The listing builds one solid part. Answer for the finished solid, in the listing's coordinates (mm). Face numbers are marked on the shaded views. A direction names the side the tool comes from. Give positions to 0.01 mm unless a question says otherwise; leave off trailing zeros. Loops run counter-clockwise (first coordinate to the right, second up) from the corner with the lowest first, then second, coordinate; pieces in that order, holes last. Notation, with made-up numbers: (-26.75, 68.5) - (31.25, 68.5) arc R7 cw to (31.25, 80.5) - close; hole circle Ø2 at (-33, -21). An arc over 180 degrees is marked (long way). Write each question's results on one line, items separated by ' | '.
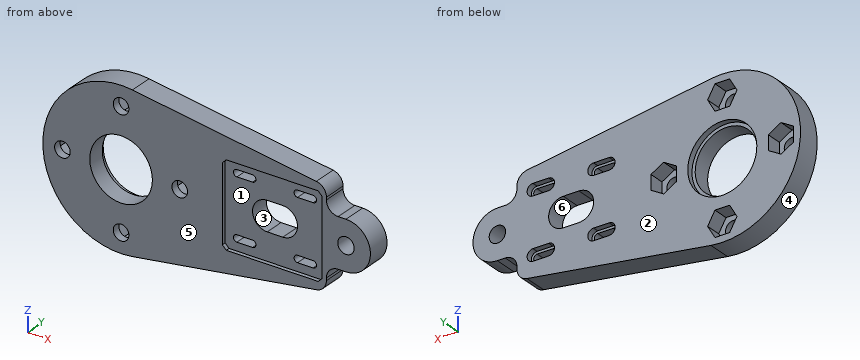
from build123d import *

# Parameters (mm, degrees)
SKETCH1_R           = 10
BOSS_EXTRUDE1_DEPTH = 12
SKETCH2_R           = 17.65
CUT_EXTRUDE1_DEPTH  = 3
CUT_EXTRUDE2_DEPTH  = 12
SKETCH4_R           = 4
CUT_EXTRUDE3_DEPTH  = 12
SKETCH5_R           = 16
CUT_EXTRUDE4_DEPTH  = 113.720894248
SKETCH6_W           = 51
SKETCH6_H           = 43
CUT_EXTRUDE5_DEPTH  = 2
CHAMFER1_SIZE       = 2
CUT_EXTRUDE6_DEPTH  = 8
CUT_EXTRUDE7_DEPTH  = 3
CUT_EXTRUDE8_DEPTH  = 7
SKETCH11_R          = 4.2
BOSS_EXTRUDE2_DEPTH = 12
FILLET1_R           = 6


with BuildPart() as part:
    # Sketch1 → Boss-Extrude1 (new body)
    with BuildSketch(Plane(origin=(0, 0, 0), x_dir=(1, 0, 0), z_dir=(0, 1, 0))):
        with BuildLine():
            Line((5.815477401, 39.574994916), (105, 25))
            Line((105, 25), (105, -25))
            Line((105, -25), (5.815477401, -39.574994916))
            ThreePointArc((5.815477401, -39.574994916), (-40, 0), (5.815477401, 39.574994916))
        make_face()
        with Locations(Location((0, 0, 0), (0, 0, 270))):
            Circle(SKETCH1_R, mode=Mode.SUBTRACT)
    extrude(amount=BOSS_EXTRUDE1_DEPTH)

    # Sketch2 → Cut-Extrude1 (cut)
    with BuildSketch(Plane(origin=(0, 12, 0), x_dir=(1, 0, 0), z_dir=(0, 1, 0))):
        with Locations(Location((0, 0, 0), (0, 0, 270))):
            Circle(SKETCH2_R)
    extrude(amount=-CUT_EXTRUDE1_DEPTH, mode=Mode.SUBTRACT)

    # Sketch3 → Cut-Extrude2 (cut)
    with BuildSketch(Plane(origin=(0, 12, 0), x_dir=(1, 0, 0), z_dir=(0, 1, 0))):
        with BuildLine():
            Line((73.3, 7.5), (81.3, 7.5))
            ThreePointArc((81.3, 7.5), (88.8, 0), (81.3, -7.5))
            Line((81.3, -7.5), (73.3, -7.5))
            ThreePointArc((73.3, -7.5), (65.8, 0), (73.3, 7.5))
        make_face()
    extrude(amount=-CUT_EXTRUDE2_DEPTH, mode=Mode.SUBTRACT)

    # Sketch4 → Cut-Extrude3 (cut)
    with BuildSketch(Plane(origin=(0, 12, 0), x_dir=(1, 0, 0), z_dir=(0, 1, 0))):
        with Locations(Location((30, 0, 0), (0, 0, 270))):
            Circle(SKETCH4_R)
        with Locations(Location((0, -30, 0), (0, 0, 270))):
            Circle(SKETCH4_R)
        with Locations(Location((-30, 0, 0), (0, 0, 270))):
            Circle(SKETCH4_R)
        with Locations(Location((0, 30, 0), (0, 0, 270))):
            Circle(SKETCH4_R)
    extrude(amount=-CUT_EXTRUDE3_DEPTH, mode=Mode.SUBTRACT)

    # Sketch5 → Cut-Extrude4 (cut, through all)
    with BuildSketch(Plane.XZ.offset(-9)):
        with Locations(Location((0, 0, 0), (0, 0, 270))):
            Circle(SKETCH5_R)
    extrude(amount=CUT_EXTRUDE4_DEPTH, mode=Mode.SUBTRACT)

    # Sketch6 → Cut-Extrude5 (cut)
    with BuildSketch(Plane.XZ):
        with Locations((77.3, 0)):
            Rectangle(SKETCH6_W, SKETCH6_H)
    extrude(amount=-CUT_EXTRUDE5_DEPTH, mode=Mode.SUBTRACT)

    # Chamfer1
    chamfer1_edges = [part.edges().sort_by_distance(p)[0] for p in [
        (102.8, 1, 21.5),
        (102.8, 1, -21.5),
        (51.8, 1, -21.5),
        (51.8, 1, 21.5),
    ]]
    chamfer(chamfer1_edges, length=CHAMFER1_SIZE)

    # Sketch7 → Cut-Extrude6 (cut)
    with BuildSketch(Plane(origin=(0, 12, 0), x_dir=(1, 0, 0), z_dir=(0, 1, 0))):
        Polygon((-7.505553499, 30), (-3.75277675, 23.5), (3.75277675, 23.5), (7.505553499, 30), (3.75277675, 36.5), (-3.75277675, 36.5), align=None)
        Polygon((-30, -7.505553499), (-23.5, -3.75277675), (-23.5, 3.75277675), (-30, 7.505553499), (-36.5, 3.75277675), (-36.5, -3.75277675), align=None)
        Polygon((30, 7.505553499), (23.5, 3.75277675), (23.5, -3.75277675), (30, -7.505553499), (36.5, -3.75277675), (36.5, 3.75277675), align=None)
        Polygon((7.505553499, -30), (3.75277675, -23.5), (-3.75277675, -23.5), (-7.505553499, -30), (-3.75277675, -36.5), (3.75277675, -36.5), align=None)
    extrude(amount=-CUT_EXTRUDE6_DEPTH, mode=Mode.SUBTRACT)

    # Sketch9 → Cut-Extrude7 (cut)
    with BuildSketch(Plane(origin=(0, 12, 0), x_dir=(1, 0, 0), z_dir=(0, 1, 0))):
        with BuildLine():
            Line((57.8, 18.5), (65.8, 18.5))
            ThreePointArc((65.8, 18.5), (68.8, 15.5), (65.8, 12.5))
            Line((65.8, 12.5), (57.8, 12.5))
            ThreePointArc((57.8, 12.5), (54.8, 15.5), (57.8, 18.5))
        make_face()
        with BuildLine():
            Line((88.8, 18.5), (96.8, 18.5))
            ThreePointArc((96.8, 18.5), (99.8, 15.5), (96.8, 12.5))
            Line((96.8, 12.5), (88.8, 12.5))
            ThreePointArc((88.8, 12.5), (85.8, 15.5), (88.8, 18.5))
        make_face()
        with BuildLine():
            Line((57.8, -12.5), (65.8, -12.5))
            ThreePointArc((65.8, -12.5), (68.8, -15.5), (65.8, -18.5))
            Line((65.8, -18.5), (57.8, -18.5))
            ThreePointArc((57.8, -18.5), (54.8, -15.5), (57.8, -12.5))
        make_face()
        with BuildLine():
            Line((88.8, -12.5), (96.8, -12.5))
            ThreePointArc((96.8, -12.5), (99.8, -15.5), (96.8, -18.5))
            Line((96.8, -18.5), (88.8, -18.5))
            ThreePointArc((88.8, -18.5), (85.8, -15.5), (88.8, -12.5))
        make_face()
    extrude(amount=-CUT_EXTRUDE7_DEPTH, mode=Mode.SUBTRACT)

    # Sketch10 → Cut-Extrude8 (cut)
    with BuildSketch(Plane(origin=(0, 9, 0), x_dir=(1, 0, 0), z_dir=(0, 1, 0))):
        with BuildLine():
            Line((57.8, 13.75), (65.8, 13.75))
            ThreePointArc((65.8, 13.75), (67.55, 15.5), (65.8, 17.25))
            Line((65.8, 17.25), (57.8, 17.25))
            ThreePointArc((57.8, 17.25), (56.05, 15.5), (57.8, 13.75))
        make_face()
        with BuildLine():
            Line((88.8, 13.75), (96.8, 13.75))
            ThreePointArc((96.8, 13.75), (98.55, 15.5), (96.8, 17.25))
            Line((96.8, 17.25), (88.8, 17.25))
            ThreePointArc((88.8, 17.25), (87.05, 15.5), (88.8, 13.75))
        make_face()
        with BuildLine():
            Line((57.8, -17.25), (65.8, -17.25))
            ThreePointArc((65.8, -17.25), (67.55, -15.5), (65.8, -13.75))
            Line((65.8, -13.75), (57.8, -13.75))
            ThreePointArc((57.8, -13.75), (56.05, -15.5), (57.8, -17.25))
        make_face()
        with BuildLine():
            Line((88.8, -17.25), (96.8, -17.25))
            ThreePointArc((96.8, -17.25), (98.55, -15.5), (96.8, -13.75))
            Line((96.8, -13.75), (88.8, -13.75))
            ThreePointArc((88.8, -13.75), (87.05, -15.5), (88.8, -17.25))
        make_face()
    extrude(amount=-CUT_EXTRUDE8_DEPTH, mode=Mode.SUBTRACT)

    # Sketch11 → Boss-Extrude2 (add)
    with BuildSketch(Plane(origin=(0, 12, 0), x_dir=(1, 0, 0), z_dir=(0, 1, 0))):
        with BuildLine():
            Line((105, -12.5), (105, 12.5))
            Line((105, 12.5), (115, 12.5))
            ThreePointArc((115, 12.5), (127.5, 0), (115, -12.5))
            Line((115, -12.5), (105, -12.5))
        make_face()
        with Locations(Location((115, 0, 0), (0, 0, 270))):
            Circle(SKETCH11_R, mode=Mode.SUBTRACT)
    extrude(amount=-BOSS_EXTRUDE2_DEPTH)

    # Fillet1
    fillet1_edges = [part.edges().sort_by_distance(p)[0] for p in [
        (105, 6, -12.5),
        (105, 6, 12.5),
        (105, 6, -25),
        (105, 6, 25),
    ]]
    fillet(fillet1_edges, radius=FILLET1_R)


solid = part.part
Item 1: For the marked faces 1, 2 and 3, determine the directions among +Z, -Z, +X, -X, +Y, -Y from which every point of the face is accessible in a straight line to the end or side of a thin tool.
Values found:
face 1: -Y | face 2: +Z, -Z, +X, -X, +Y | face 3: +Y, -Y
Item 2: For a pull along Z with two mould halves and no side action, classify the marked faces 4, 5 and 6 as released by +Z, released by -Z, zero draft, split by the parting line, or undercut.
Values found:
face 4: split by the parting line | face 5: zero draft | face 6: undercut
Item 3: A cutting plane is placed at B-B, the plane z = -28. Determine the outline of the cut face in (x, y).
Values found:
outline: (-28.57, 0) - (-3.46, 0) - (-3.46, 4) - (-6.35, 4) - (-6.35, 12) - (-28.57, 12) - close; (3.46, 0) - (84.58, 0) - (84.58, 12) - (6.35, 12) - (6.35, 4) - (3.46, 4) - close
Item 4: Flat-ended cylindrical pins translate along their axes: P1, Ø14.5, axis at x = 3.5, z = 29, coming from the +Y side; P2, Ø1.5, axis at y = 9, z = -7.5, coming from the +X side; P3, Ø10.5, axis at x = -4, z = -7.5, coming from the +Y side; P4, Ø4.5, axis at x = 112.5, y = 8, coming from the -Z side. Find the tip coordinate at first contact, or state that the pin passes through.
Values found:
P1: stops at y = 12 | P2: stops at x = 125.52 | P3: passes through | P4: stops at z = -12.55
Item 5: A cutting plane is placed at C-C, the plane x = 32.5. Determine the outline of the cut face in (y, z).
Values found:
outline: (0, -35.65) - (12, -35.65) - (12, -6.06) - (4, -6.06) - (4, -3.12) - (0, -3.12) - close; (0, 3.12) - (4, 3.12) - (4, 6.06) - (12, 6.06) - (12, 35.65) - (0, 35.65) - close
Item 6: A cutting plane is placed at A-A, the plane x = 0. Determine the outline of the cut face in (y, z).
Values found:
outline: (0, -40) - (12, -40) - (12, -36.5) - (4, -36.5) - (4, -34) - (0, -34) - close; (0, -26) - (4, -26) - (4, -23.5) - (12, -23.5) - (12, -17.65) - (9, -17.65) - (9, -16) - (0, -16) - close; (0, 16) - (9, 16) - (9, 17.65) - (12, 17.65) - (12, 23.5) - (4, 23.5) - (4, 26) - (0, 26) - close; (0, 34) - (4, 34) - (4, 36.5) - (12, 36.5) - (12, 40) - (0, 40) - close
Item 7: Find the intervals of material crossed by line 1 along X through (y, z) = (1.8, 0); line 2 along X through (y, z) = (2.4, 0); line 3 along Z through (x, y) = (113.5, 3.25), in increasing order. Write a range as [from, to].
Values found:
line 1: x = [-40, -34], [-26, -16], [16, 26], [34, 51.8], [102.8, 110.8], [119.2, 127.5] | line 2: x = [-40, -34], [-26, -16], [16, 26], [34, 65.8], [88.8, 110.8], [119.2, 127.5] | line 3: z = [-12.5, -3.92], [3.92, 12.5]
Item 8: A cutting plane is placed at D-D, the plane y = 10.5. Count the separate pieces of the cut face and the enclosed holes in it, plus the area to 3 significant figures.
Values found:
separate pieces: 1 | enclosed holes: 11 | area: 7,660 mm²
